from build123d import *

# Parameters (mm, degrees)
CROQUIS1_R                   = 15
SALIENTE_EXTRUIR1_DEPTH      = 160
CROQUIS2_R                   = 15
CROQUIS2_R_2                 = 5
CORTAR_EXTRUIR_L_MINA1_DEPTH = 40
CORTAR_EXTRUIR_L_MINA2_START = -40
CROQUIS3_R                   = 15
CROQUIS3_R_2                 = 5
CORTAR_EXTRUIR_L_MINA2_DEPTH = 40


with BuildPart() as part:
    # Croquis1 → Saliente-Extruir1 (new body)
    with BuildSketch(Plane.XY):
        Circle(CROQUIS1_R)
    extrude(amount=SALIENTE_EXTRUIR1_DEPTH)

    # Croquis2 → Cortar-Extruir-Lámina1 (cut)
    with BuildSketch(Plane(origin=(0, 0, 0), x_dir=(-1, 0, 0), z_dir=(0, 0, -1))):
        Circle(CROQUIS2_R)
        Circle(CROQUIS2_R_2, mode=Mode.SUBTRACT)
    extrude(amount=-CORTAR_EXTRUIR_L_MINA1_DEPTH, mode=Mode.SUBTRACT)

    # Croquis3 → Cortar-Extruir-Lámina2 (cut)
    with BuildSketch(Plane.XY.offset(160).offset(CORTAR_EXTRUIR_L_MINA2_START)):
        Circle(CROQUIS3_R)
        Circle(CROQUIS3_R_2, mode=Mode.SUBTRACT)
    extrude(amount=CORTAR_EXTRUIR_L_MINA2_DEPTH, mode=Mode.SUBTRACT)


solid = part.part
Build history of the part. All positions in model axes, mm. A direction names the side the tool comes from. Round coordinates to 2 decimals unless told otherwise and drop trailing zeros. Write each loop counter-clockwise with the first axis right and the second up, starting at its lowest first coordinate (ties: lowest second). Pieces come first, ordered by that corner, then holes. Notation, with made-up numbers: (56.5, -11.75) -> (104.5, -11.75) arc R30 ccw to (104.5, 15.25) -> close; hole circle Ø2 at (16, -6.75). An arc over 180 degrees is marked (long way). Use one line per item in the form item = value.
Q1. Drill centre lines: L1, parallel to Z at x = 11.5, y = -7.25; L2, parallel to Y at x = 0.5, z = 45.5; L3, parallel to Y at x = 2.75, z = 39.5. Where is each one in solid material? Low to high.
Conclusion:
L1 = 40 to 120
L2 = -14.99 to 14.99
L3 = -4.18 to 4.18
Q2. Band-saw the part on C-C, the plane z = 53. Write the cut outline in (x, y), then the cut area to 3 significant figures.
Conclusion:
outline = circle Ø30 at (0, 0)
area = 707 mm²
Q3. Drop flat-ended pins along their axis: P1, Ø3, axis at x = 2, z = 30, coming from the +Y side; P2, Ø3, axis at x = 0.5, y = -10, coming from the -Z side; P3, Ø4, axis at y = -9.5, z = 84.5, coming from the -X side. Give the stop position or say it passes through.
Conclusion:
P1 = 4.97
P2 = 40
P3 = -12.99
Q4. Tool access for faces 1 (the flat face through (0, 0, 160)), 2 (the cylindrical face through (-1.08, -4.88, 139.72)), 3 (the cylindrical face through (1.08, -4.88, 19.72)): list every direction of +Z, -Z, +X, -X, +Y, -Y with a clear straight run to the whole face (end or side of a thin tool).
Conclusion:
face_1 = +Z, +X, -X, +Y, -Y
face_2 = +Z
face_3 = -Z
Q5. Band-saw the part on D-D, the plane x = 9. Write the cut outline in (y, z), then the cut area to 3 significant figures.
Conclusion:
outline = (-12, 40) -> (12, 40) -> (12, 120) -> (-12, 120) -> close
area = 1,920 mm²
Q6. Band-saw the part on A-A, the plane y = 0. Write the cut outline in (x, z).
Conclusion:
outline = (-15, 40) -> (-5, 40) -> (-5, 0) -> (5, 0) -> (5, 40) -> (15, 40) -> (15, 120) -> (5, 120) -> (5, 160) -> (-5, 160) -> (-5, 120) -> (-15, 120) -> close
